Print and shaded views of the part. All mm, measured from the part's lowest x, y and z. Round coordinates to 2 decimals unless told otherwise and drop trailing zeros. Write each loop counter-clockwise with the first axis right and the second up, starting at its lowest first coordinate (ties: lowest second). Pieces come first, ordered by that corner, then holes. Notation, with made-up numbers: (-27.5, 82) - (-19.5, 82) arc R28 cw to (-19.5, 111) - close; hole circle Ø7 at (37.25, 44). An arc over 180 degrees is marked (long way). Answer as a JSON object with one key per item and string values. Group by question number.
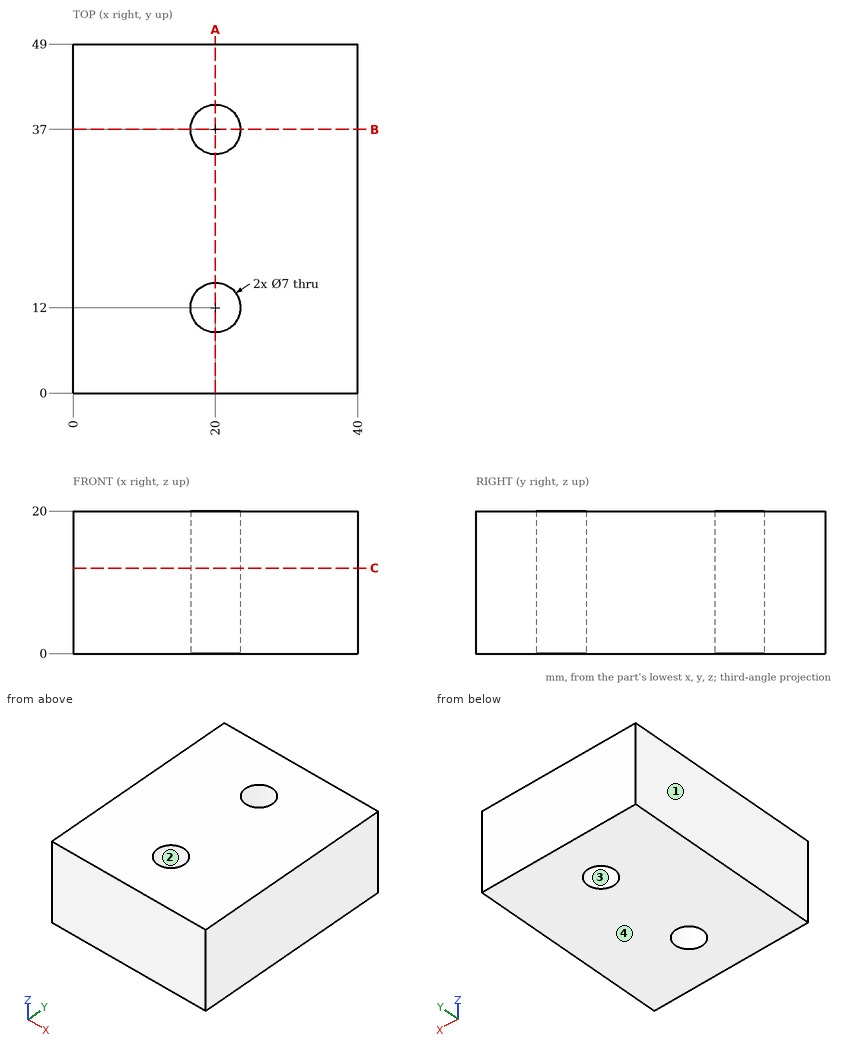
(1) Slice it at B-B (y = 37). Write the cut outline in (x, z).
(2) Slice it at C-C (z = 12). Write the cut outline in (x, y), then the cut area to 3 significant figures.
(3) Slice it at A-A (x = 20). Write the cut outline in (y, z), then the cut area to 3 significant figures.
(4) Pull direction X, two halves, no side cores. Call the marked faces 1, 2, 3 and 4: pulls with the +X half, pulls with the -X half, needs draft (parallel to the pull), parting line crosses it, or undercut.
(5) Drill centre lines: line 1 (Y direction, x = 20, z = 6.75); line 2 (X direction, y = 11, z = 15.5); line 3 (X direction, y = 39, z = 8). Where is each one in solid material? Low to high. Write a range as from..to.
Answer:
{
 "1": {"outline": "(0, 0) - (16.5, 0) - (16.5, 20) - (0, 20) - close; (23.5, 0) - (40, 0) - (40, 20) - (23.5, 20) - close"},
 "2": {"outline": "(0, 0) - (40, 0) - (40, 49) - (0, 49) - close; hole circle Ø7 at (20, 12); hole circle Ø7 at (20, 37)", "area": "1,880 mm²"},
 "3": {"outline": "(0, 0) - (8.5, 0) - (8.5, 20) - (0, 20) - close; (15.5, 0) - (33.5, 0) - (33.5, 20) - (15.5, 20) - close; (40.5, 0) - (49, 0) - (49, 20) - (40.5, 20) - close", "area": "700 mm²"},
 "4": {"face 1": "pulls with the -X half", "face 2": "undercut", "face 3": "undercut", "face 4": "needs draft"},
 "5": {"line 1": "0..8.5, 15.5..33.5, 40.5..49", "line 2": "0..16.65, 23.35..40", "line 3": "0..17.13, 22.87..40"}
}
